from build123d import *

# Parameters (mm, degrees)
BOSS_EXTRUDE1_DEPTH = 15
SKETCH5_W           = 5
SKETCH5_H           = 60
SKETCH5_W_2         = 125
SKETCH5_H_2         = 5
CUT_EXTRUDE2_DEPTH  = 5


with BuildPart() as part:
    # Sketch1 → Boss-Extrude1 (new body)
    with BuildSketch(Plane(origin=(0, 0, 0), x_dir=(1, 0, 0), z_dir=(0, 1, 0))):
        Polygon((-105, 48), (-105, 50), (-103, 50), (103, 50), (105, 50), (105, 48), (105, -48), (105, -50), (103, -50), (-103, -50), (-105, -50), (-105, -48), align=None)
    extrude(amount=BOSS_EXTRUDE1_DEPTH)

    # Sketch5 → Cut-Extrude2 (cut)
    with BuildSketch(Plane(origin=(0, 15, 0), x_dir=(1, 0, 0), z_dir=(0, 1, 0))):
        with Locations((100, 0)):
            Rectangle(SKETCH5_W, SKETCH5_H)
        with Locations((-100, 0)):
            Rectangle(SKETCH5_W, SKETCH5_H)
        with Locations((0, -45)):
            Rectangle(SKETCH5_W_2, SKETCH5_H_2)
        with Locations((0, 45)):
            Rectangle(SKETCH5_W_2, SKETCH5_H_2)
    extrude(amount=-CUT_EXTRUDE2_DEPTH, mode=Mode.SUBTRACT)


solid = part.part
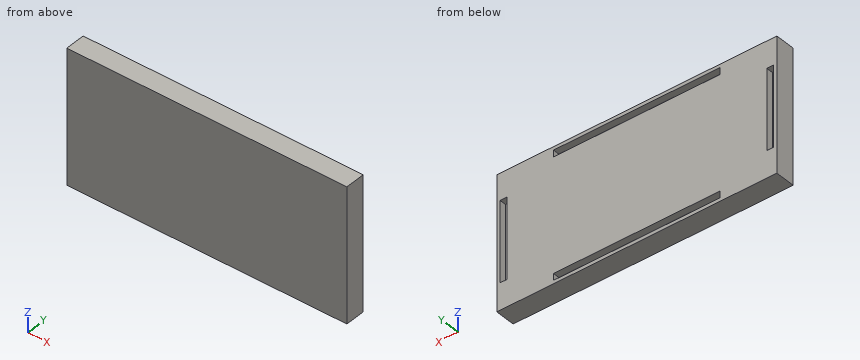
The listing builds one solid part. Answer for the finished solid, in the listing's coordinates (mm). Give positions to 0.01 mm unless a question says otherwise; leave off trailing zeros. Write each loop counter-clockwise with the first axis right and the second up, starting at its lowest first coordinate (ties: lowest second). Pieces come first, ordered by that corner, then holes. Notation, with made-up numbers: (79, -2) -> (120, -2) arc R7 ccw to (120, 6) -> close; hole circle Ø10 at (-36, 0). An arc over 180 degrees is marked (long way). Use a Markdown table: item, result.
(1) Section A-A, the plane z = -22 is taken. Determine the outline of the cut face in (x, y).
Return value:
| item | result |
|---|---|
| outline | (-105, 0) -> (105, 0) -> (105, 15) -> (102.5, 15) -> (102.5, 10) -> (97.5, 10) -> (97.5, 15) -> (-97.5, 15) -> (-97.5, 10) -> (-102.5, 10) -> (-102.5, 15) -> (-105, 15) -> close |
(2) Section B-B, the plane x = -37.5 is taken. Determine the outline of the cut face in (y, z), then the cut area to 3 significant figures.
Return value:
| item | result |
|---|---|
| outline | (0, -50) -> (15, -50) -> (15, -47.5) -> (10, -47.5) -> (10, -42.5) -> (15, -42.5) -> (15, 42.5) -> (10, 42.5) -> (10, 47.5) -> (15, 47.5) -> (15, 50) -> (0, 50) -> close |
| area | 1,450 mm2 |
(3) Find the intervals of material crossed by probe 1 along Z at (x, y) = (-27, 13.5); probe 2 along X at (y, z) = (10.25, 26); probe 3 along X at (y, z) = (13, -44), in increasing order. Write a range as from..to.
Return value:
| item | result |
|---|---|
| probe 1 | -50..-47.5, -42.5..42.5, 47.5..50 |
| probe 2 | -105..-102.5, -97.5..97.5, 102.5..105 |
| probe 3 | -105..-62.5, 62.5..105 |
